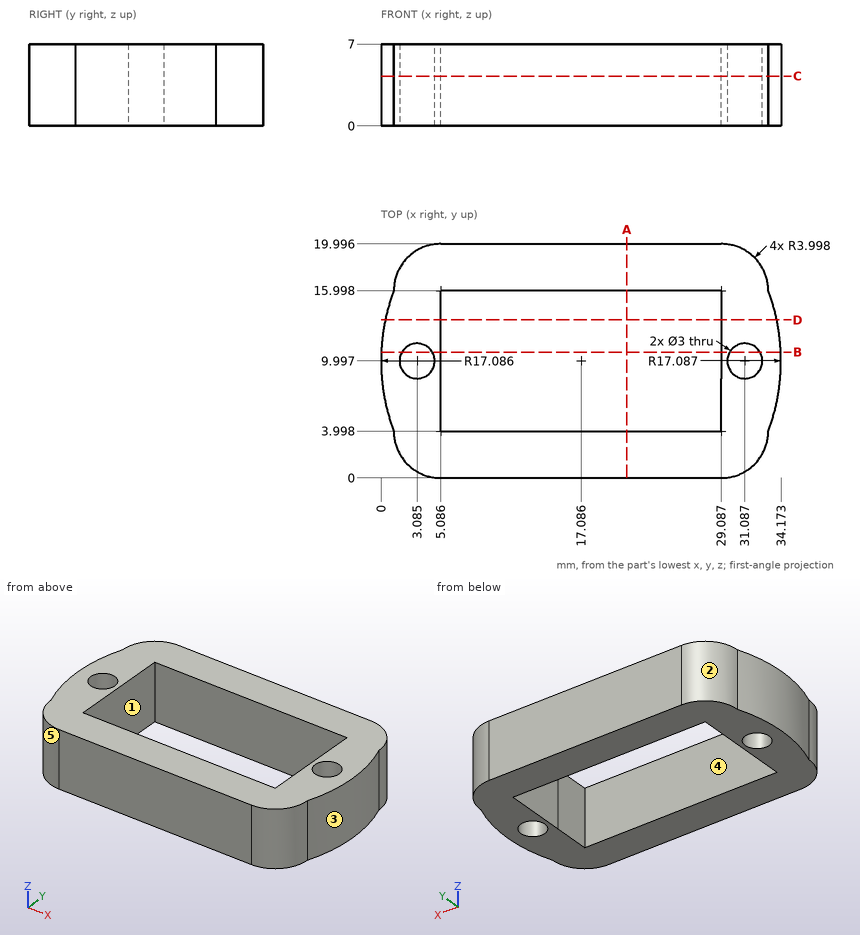
Source: three-view drawing plus pictorial views. Frame: mm from the lowest corner of the part. A direction names the side the tool comes from. Give positions to 0.01 mm unless a question says otherwise; leave off trailing zeros. Write each loop counter-clockwise with the first axis right and the second up, starting at its lowest first coordinate (ties: lowest second). Pieces come first, ordered by that corner, then holes.
(1) Ray query, line 1 (Y direction, x = 29, z = 1) (1 decimal); line 2 (X direction, y = 6.5, z = 2) (1 decimal); line 3 (X direction, y = 15.25, z = 0.75) (1 decimal). Return the intervals inside material, ascending.
(2) Cut plane C-C, the plane z = 4.25. Return loops of the section in (x, y) (1 decimal).
(3) First-contact query: P1, Ø3, axis at y = 5.5, z = 1.5, coming from the +X side; P2, Ø1.5, axis at y = 14.5, z = 4.5, coming from the +X side (1 decimal); P3, Ø1.3, axis at y = 7, z = 3.5, coming from the -X side. Flat tips, straight axial feed; report the tip coordinate or a pass-through.
(4) Cut plane A-A, the plane x = 21. Return loops of the section in (y, z) (1 decimal).
(5) Cut plane B-B, the plane y = 10.75. Return loops of the section in (x, z).
(6) Access query for the marked faces 4 and 5. Directions: +Z, -Z, +X, -X, +Y, -Y. A direction counts if a zero-diameter tool reaches every point of the face in a straight line with its end or side. Return the directions, or none.
(7) Mould query, pull axis X, two halves, no side actions, for the marked faces 1, 2 and 3. Classes: released by +X, released by -X, zero draft, split by the parting line, or undercut.
(8) Cut plane D-D, the plane y = 13.5. Return loops of the section in (x, z).
Values follow:
1. line 1: y = 0 to 4, 16 to 20
1. line 2: x = 0.4 to 5.1, 29.1 to 33.8
1. line 3: x = 0.8 to 5.1, 29.1 to 33.3
2. outline: (1.1, 4) arc R4 ccw to (5.1, 0) - (29.1, 0) arc R4 ccw to (33.1, 4) arc R17.1 ccw to (33.1, 16) arc R4 ccw to (29.1, 20) - (5.1, 20) arc R4 ccw to (1.1, 16) arc R17.1 ccw to start; hole circle Ø3 at (3.1, 10); hole (5.1, 4) - (29.1, 4) - (29.1, 8.5) - (29.1, 16) - (5.1, 16) - close; hole circle Ø3 at (31.1, 10)
3. P1: stops at x = 33.91
3. P2: stops at x = 33.8
3. P3: stops at x = 0.16
4. outline: (0, 0) - (4, 0) - (4, 7) - (0, 7) - close; (16, 0) - (20, 0) - (20, 7) - (16, 7) - close
5. outline: (0.02, 0) - (1.79, 0) - (1.79, 7) - (0.02, 7) - close; (4.38, 0) - (5.09, 0) - (5.09, 7) - (4.38, 7) - close; (29.09, 0) - (29.79, 0) - (29.79, 7) - (29.09, 7) - close; (32.38, 0) - (34.16, 0) - (34.16, 7) - (32.38, 7) - close
6. face 4: +Z, -Z
6. face 5: +Z, -Z, -X, -Y
7. face 1: undercut
7. face 2: released by -X
7. face 3: released by +X
8. outline: (0.36, 0) - (5.09, 0) - (5.09, 7) - (0.36, 7) - close; (29.09, 0) - (33.81, 0) - (33.81, 7) - (29.09, 7) - close
